```python
from build123d import *

# Parameters (mm, degrees)
SKETCH1_W                       = 46
SKETCH1_H                       = 137
BOSS_EXTRUDE1_DEPTH             = 25
FILLET1_R                       = 2
SKETCH2_R                       = 0.825
SKETCH2_R_2                     = 2.45
BOSS_EXTRUDE4_DEPTH             = 5
BOSS_EXTRUDE4_DIRECTION_2_REACH = 143.149


with BuildPart() as part:
    # Sketch1 → Boss-Extrude1 (new body)
    with BuildSketch(Plane.XY):
        with Locations((0, 68.5)):
            Rectangle(SKETCH1_W, SKETCH1_H)
    extrude(amount=BOSS_EXTRUDE1_DEPTH)

    # Fillet1
    fillet1_edges = [part.edges().sort_by_distance(p)[0] for p in [
        (23, 68.5, 25),
        (0, 137, 25),
        (-23, 68.5, 25),
        (0, 137, 0),
        (23, 68.5, 0),
        (0, 0, 0),
        (-23, 68.5, 0),
        (-23, 137, 12.5),
        (23, 137, 12.5),
        (23, 0, 12.5),
        (-23, 0, 12.5),
        (0, 0, 25),
    ]]
    fillet(fillet1_edges, radius=FILLET1_R)

    # Sketch2 → Boss-Extrude4 (add)
    with BuildSketch(Plane(origin=(0, 0, 0), x_dir=(-1, 0, 0), z_dir=(0, 0, -1))):
        with Locations((-16.666666667, 135)):
            Circle(SKETCH2_R)
        with Locations((-15, 135)):
            Circle(SKETCH2_R)
        with Locations((-13.333333333, 135)):
            Circle(SKETCH2_R)
        with Locations((13, 134.55)):
            Circle(SKETCH2_R_2)
        with Locations((18, 134.55)):
            Circle(SKETCH2_R_2)
    extrude(amount=BOSS_EXTRUDE4_DEPTH)

    # Sketch2 → Boss-Extrude4 direction 2 (add, up to next)
    with BuildSketch(Plane(origin=(0, 0, 0), x_dir=(-1, 0, 0), z_dir=(0, 0, -1)), mode=Mode.PRIVATE) as boss_extrude4_direction_2_sk1:
        with Locations((-16.666666667, 135)):
            Circle(SKETCH2_R)
    boss_extrude4_direction_2_tool1 = extrude(boss_extrude4_direction_2_sk1.sketch, amount=-BOSS_EXTRUDE4_DIRECTION_2_REACH, mode=Mode.PRIVATE) - part.part
    # Sketch2 → Boss-Extrude4 direction 2 (add, up to next)
    with BuildSketch(Plane(origin=(0, 0, 0), x_dir=(-1, 0, 0), z_dir=(0, 0, -1)), mode=Mode.PRIVATE) as boss_extrude4_direction_2_sk2:
        with Locations((-15, 135)):
            Circle(SKETCH2_R)
    boss_extrude4_direction_2_tool2 = extrude(boss_extrude4_direction_2_sk2.sketch, amount=-BOSS_EXTRUDE4_DIRECTION_2_REACH, mode=Mode.PRIVATE) - part.part
    # Sketch2 → Boss-Extrude4 direction 2 (add, up to next)
    with BuildSketch(Plane(origin=(0, 0, 0), x_dir=(-1, 0, 0), z_dir=(0, 0, -1)), mode=Mode.PRIVATE) as boss_extrude4_direction_2_sk3:
        with Locations((-13.333333333, 135)):
            Circle(SKETCH2_R)
    boss_extrude4_direction_2_tool3 = extrude(boss_extrude4_direction_2_sk3.sketch, amount=-BOSS_EXTRUDE4_DIRECTION_2_REACH, mode=Mode.PRIVATE) - part.part
    # Sketch2 → Boss-Extrude4 direction 2 (add, up to next)
    with BuildSketch(Plane(origin=(0, 0, 0), x_dir=(-1, 0, 0), z_dir=(0, 0, -1)), mode=Mode.PRIVATE) as boss_extrude4_direction_2_sk4:
        with Locations((13, 134.55)):
            Circle(SKETCH2_R_2)
    boss_extrude4_direction_2_tool4 = extrude(boss_extrude4_direction_2_sk4.sketch, amount=-BOSS_EXTRUDE4_DIRECTION_2_REACH, mode=Mode.PRIVATE) - part.part
    # Sketch2 → Boss-Extrude4 direction 2 (add, up to next)
    with BuildSketch(Plane(origin=(0, 0, 0), x_dir=(-1, 0, 0), z_dir=(0, 0, -1)), mode=Mode.PRIVATE) as boss_extrude4_direction_2_sk5:
        with Locations((18, 134.55)):
            Circle(SKETCH2_R_2)
    boss_extrude4_direction_2_tool5 = extrude(boss_extrude4_direction_2_sk5.sketch, amount=-BOSS_EXTRUDE4_DIRECTION_2_REACH, mode=Mode.PRIVATE) - part.part
    add(boss_extrude4_direction_2_tool1.solids().sort_by_distance((16.666667, 135, 0))[0])
    add(boss_extrude4_direction_2_tool2.solids().sort_by_distance((15, 135, 0))[0])
    add(boss_extrude4_direction_2_tool3.solids().sort_by_distance((13.333333, 135, 0))[0])
    add(boss_extrude4_direction_2_tool4.solids().sort_by_distance((-13, 134.55, 0))[0])
    add(boss_extrude4_direction_2_tool5.solids().sort_by_distance((-18, 134.55, 0))[0])


solid = part.part
```
The listing builds one solid part. Answer for the finished solid, in the listing's coordinates (mm). Round coordinates to 2 decimals unless told otherwise and drop trailing zeros. Order: outer loops, then holes, each group sorted by start corner. A loop starts at its lowest first (then second) coordinate and runs counter-clockwise, first axis right, second up. Notation, with made-up numbers: (37, -8.75) - (77, -8.75) arc R36 cw to (77, 29.25) - close; hole circle Ø11 at (-8, -21). An arc over 180 degrees is marked (long way). Put each result on its own line as item: value. Start each with the question number.
(1) Find section B-B (x = 1.5). Give the vertices of the cut face in (y, z).
(2) Straight lines are drawn through the part: probe 1 along Z at (x, y) = (-6, 62.5); probe 2 along Y at (x, z) = (-17, 23.5); probe 3 along X at (y, z) = (123.5, 23.75). For each, find the intervals that lie inside material, in ascending order. Write a range as from..to.
(3) Given P1, Ø1.5, axis at x = -15.5, y = 115.5, coming from the -Z side; P2, Ø6, axis at y = 77, z = -1.5, coming from the -X side; P3, Ø5, axis at x = -4.5, z = 16, coming from the -Y side, each flat-ended and moving along its own axis, determine where each tip first touches the part or whether it passes through.
(4) Find section A-A (y = 34.5). Give the vertices of the cut face in (x, z), plus the area to 3 significant figures.
Reply:
1. outline: (0, 2) arc R2 ccw to (2, 0) - (135, 0) arc R2 ccw to (137, 2) - (137, 23) arc R2 ccw to (135, 25) - (2, 25) arc R2 ccw to (0, 23) - close
2. probe 1: 0..25
2. probe 2: 0.06..136.94
2. probe 3: -22.85..22.85
3. P1: z = 0
3. P2: x = -22.94
3. P3: y = 0
4. outline: (-23, 2) arc R2 ccw to (-21, 0) - (21, 0) arc R2 ccw to (23, 2) - (23, 23) arc R2 ccw to (21, 25) - (-21, 25) arc R2 ccw to (-23, 23) - close
4. area: 1,150 mm^2
